from build123d import *

# Parameters (mm, degrees)
F0_W     = 167.0182794333
F0_H     = 48.4514534473
F1_DEPTH = 42.8443159908
F2_DEPTH = 10.226784274
F3_W     = 92.7675813437
F3_H     = 58.6782377213
F4_DEPTH = 38.0648057908


with BuildPart() as f1:
    # F0 (on Top) → F1 (new body)
    with BuildSketch(Plane.XY):
        with Locations((9.258441627, -0.4500597715)):
            Rectangle(F0_W, F0_H)
    extrude(amount=F1_DEPTH)

    # F2 (add): a face of the model
    f2_faces = [f1.faces().sort_by_distance(p)[0] for p in [
        (9.258441627, -24.6757864952, 21.4221579954),
    ]]
    extrude(f2_faces, amount=F2_DEPTH)

    # F3 (on face) → F4 (join)
    with BuildSketch(Plane.XY.offset(42.8443159908)):
        with Locations((46.3837906718, -5.5634519085)):
            Rectangle(F3_W, F3_H)
    extrude(amount=F4_DEPTH)


solid = f1.part
Geometry: final body of the model. Coordinates: model frame, mm. A direction names the side the tool comes from. Give positions to 0.01 mm unless a question says otherwise; leave off trailing zeros. Loops run counter-clockwise (first coordinate to the right, second up) from the corner with the lowest first, then second, coordinate; pieces in that order, holes last. Notation, with made-up numbers: (-13.75, -39.75) - (42.25, -39.75) arc R28 cw to (42.25, -13.75) - close; hole circle Ø10 at (76.5, 71.25). An arc over 180 degrees is marked (long way). One line per question, with ' | ' between items. Start each with the question number.
(1) Reachability of faces 1 (the flat face through (0, -6, 62)), 2 (the flat face through (8, -5, 0)) from +Z, -Z, +X, -X, +Y, -Y: full face, straight path, thin tool, end or side. Return the list, or none.
(2) Section query C-C on x = -53.5. Return loops of the section in (y, z), then the cut area to 3 significant figures.
(3) Section query A-A on y = -14. Return loops of the section in (x, z), then the cut area to 3 significant figures.
(4) Ray query, line 1 (Z direction, x = -29.5, y = -22.5); line 2 (X direction, y = -12, z = 73). Return the intervals inside material, ascending. Write a range as from..to.
(5) Section query B-B on z = 60. Return loops of the section in (x, y).
(6) Contact query for a flat-ended pin moving along its axis: pin 1 (12 mm diameter, centred on y = -10, z = 71, fed in from -X). Output: stop coordinate, or through.
The answers:
1) face 1: +Z, -X, +Y, -Y | face 2: -Z, +X, -X, +Y, -Y
2) outline: (-34.9, 0) - (23.78, 0) - (23.78, 42.84) - (-34.9, 42.84) - close | area: 2,510 mm2
3) outline: (-74.25, 0) - (92.77, 0) - (92.77, 80.91) - (0, 80.91) - (0, 42.84) - (-74.25, 42.84) - close | area: 10,700 mm2
4) line 1: 0..42.84 | line 2: 0..92.77
5) outline: (0, -34.9) - (92.77, -34.9) - (92.77, 23.78) - (0, 23.78) - close
6) pin 1: x = 0
